```python
from build123d import *

# Parameters (mm, degrees)
SKETCH1_W           = 100
SKETCH1_H           = 40
BOSS_EXTRUDE1_DEPTH = 38
CUT_EXTRUDE2_START  = -12
SKETCH2_W           = 39.5
SKETCH2_H           = 34
CUT_EXTRUDE2_DEPTH  = 21
CUT_EXTRUDE3_DEPTH  = 9
CUT_EXTRUDE4_REACH  = 81.36
SKETCH4_R           = 1.45
SKETCH5_W           = 100
SKETCH5_H           = 19
CUT_EXTRUDE5_DEPTH  = 87.215210375
FILLET1_R           = 0.5
CUT_EXTRUDE11_REACH = 73.063
SKETCH10_R          = 3.5


with BuildPart() as part:
    # Sketch1 → Boss-Extrude1 (new body)
    with BuildSketch(Plane.XY):
        with Locations((16.25, 1.5625)):
            Rectangle(SKETCH1_W, SKETCH1_H)
    extrude(amount=BOSS_EXTRUDE1_DEPTH)

    # Sketch2 → Cut-Extrude2 (cut)
    with BuildSketch(Plane(origin=(0, 0, 0), x_dir=(-1, 0, 0), z_dir=(0, 0, -1)).offset(CUT_EXTRUDE2_START)):
        with Locations((-38.5, 1.5625)):
            Rectangle(SKETCH2_W, SKETCH2_H)
        with Locations((6, 1.5625)):
            Rectangle(SKETCH2_W, SKETCH2_H)
    extrude(amount=-CUT_EXTRUDE2_DEPTH, mode=Mode.SUBTRACT)

    # Sketch3 → Cut-Extrude3 (cut)
    with BuildSketch(Plane(origin=(-3.362318072, 0, 0), x_dir=(-1, 0, 0), z_dir=(0, 0, -1))):
        with BuildLine():
            ThreePointArc((-61.593370612, 1.614325749), (-20.676836723, -17.421621422), (21.715969185, -1.949710178))
            ThreePointArc((21.715969185, -1.949710178), (22.204299442, 9.465009595), (10.78957967, 9.953339852))
            ThreePointArc((10.78957967, 9.953339852), (-19.986233449, -1.278769909), (-49.690320582, 12.540715264))
            ThreePointArc((-49.690320582, 12.540715264), (-61.105040355, 13.029045522), (-61.593370612, 1.614325749))
        make_face()
    extrude(amount=-CUT_EXTRUDE3_DEPTH, mode=Mode.SUBTRACT)

    # Sketch4 → Cut-Extrude4 (cut, up to next)
    with BuildSketch(Plane(origin=(0, 0, 0), x_dir=(-1, 0, 0), z_dir=(0, 0, -1)), mode=Mode.PRIVATE) as cut_extrude4_sk1:
        with Locations((-62.25, 16.0625)):
            Circle(SKETCH4_R)
    cut_extrude4_tool1 = extrude(cut_extrude4_sk1.sketch, amount=-CUT_EXTRUDE4_REACH, mode=Mode.PRIVATE) & part.part
    # Sketch4 → Cut-Extrude4 (cut, up to next)
    with BuildSketch(Plane(origin=(0, 0, 0), x_dir=(-1, 0, 0), z_dir=(0, 0, -1)), mode=Mode.PRIVATE) as cut_extrude4_sk2:
        with Locations((-62.25, -12.9375)):
            Circle(SKETCH4_R)
    cut_extrude4_tool2 = extrude(cut_extrude4_sk2.sketch, amount=-CUT_EXTRUDE4_REACH, mode=Mode.PRIVATE) & part.part
    # Sketch4 → Cut-Extrude4 (cut, up to next)
    with BuildSketch(Plane(origin=(0, 0, 0), x_dir=(-1, 0, 0), z_dir=(0, 0, -1)), mode=Mode.PRIVATE) as cut_extrude4_sk3:
        with Locations((29.75, 16.0625)):
            Circle(SKETCH4_R)
    cut_extrude4_tool3 = extrude(cut_extrude4_sk3.sketch, amount=-CUT_EXTRUDE4_REACH, mode=Mode.PRIVATE) & part.part
    # Sketch4 → Cut-Extrude4 (cut, up to next)
    with BuildSketch(Plane(origin=(0, 0, 0), x_dir=(-1, 0, 0), z_dir=(0, 0, -1)), mode=Mode.PRIVATE) as cut_extrude4_sk4:
        with Locations((29.75, -12.9375)):
            Circle(SKETCH4_R)
    cut_extrude4_tool4 = extrude(cut_extrude4_sk4.sketch, amount=-CUT_EXTRUDE4_REACH, mode=Mode.PRIVATE) & part.part
    add(cut_extrude4_tool1.solids().sort_by_distance((62.25, 16.0625, 0))[0], mode=Mode.SUBTRACT)
    add(cut_extrude4_tool2.solids().sort_by_distance((62.25, -12.9375, 0))[0], mode=Mode.SUBTRACT)
    add(cut_extrude4_tool3.solids().sort_by_distance((-29.75, 16.0625, 0))[0], mode=Mode.SUBTRACT)
    add(cut_extrude4_tool4.solids().sort_by_distance((-29.75, -12.9375, 0))[0], mode=Mode.SUBTRACT)

    # Sketch5 → Cut-Extrude5 (cut, through all)
    with BuildSketch(Plane(origin=(0, 21.5625, 0), x_dir=(1, 0, 0), z_dir=(0, 1, 0))):
        with Locations((16.25, -9.5)):
            Rectangle(SKETCH5_W, SKETCH5_H)
    extrude(amount=-CUT_EXTRUDE5_DEPTH, mode=Mode.SUBTRACT)

    # Fillet1
    fillet1_edges = [part.edges().sort_by_distance(p)[0] for p in [
        (58.25, 18.5625, 26),
        (18.75, 18.5625, 26),
        (18.75, -15.4375, 26),
        (58.25, -15.4375, 26),
        (13.75, 18.5625, 26),
        (-25.75, 18.5625, 26),
        (-25.75, -15.4375, 26),
        (13.75, -15.4375, 26),
    ]]
    fillet(fillet1_edges, radius=FILLET1_R)

    # Sketch10 → Cut-Extrude11 (cut, up to next)
    with BuildSketch(Plane(origin=(0, 0, 33), x_dir=(-1, 0, 0), z_dir=(0, 0, -1)), mode=Mode.PRIVATE) as cut_extrude11_sk1:
        with Locations((-49.860388068, -8.232477434)):
            Circle(SKETCH10_R)
    cut_extrude11_tool1 = extrude(cut_extrude11_sk1.sketch, amount=-CUT_EXTRUDE11_REACH, mode=Mode.PRIVATE) & part.part
    # Sketch10 → Cut-Extrude11 (cut, up to next)
    with BuildSketch(Plane(origin=(0, 0, 33), x_dir=(-1, 0, 0), z_dir=(0, 0, -1)), mode=Mode.PRIVATE) as cut_extrude11_sk2:
        with Locations((-27.139611932, 11.357477434)):
            Circle(SKETCH10_R)
    cut_extrude11_tool2 = extrude(cut_extrude11_sk2.sketch, amount=-CUT_EXTRUDE11_REACH, mode=Mode.PRIVATE) & part.part
    # Sketch10 → Cut-Extrude11 (cut, up to next)
    with BuildSketch(Plane(origin=(0, 0, 33), x_dir=(-1, 0, 0), z_dir=(0, 0, -1)), mode=Mode.PRIVATE) as cut_extrude11_sk3:
        with Locations((-5.360388068, -8.232477434)):
            Circle(SKETCH10_R)
    cut_extrude11_tool3 = extrude(cut_extrude11_sk3.sketch, amount=-CUT_EXTRUDE11_REACH, mode=Mode.PRIVATE) & part.part
    # Sketch10 → Cut-Extrude11 (cut, up to next)
    with BuildSketch(Plane(origin=(0, 0, 33), x_dir=(-1, 0, 0), z_dir=(0, 0, -1)), mode=Mode.PRIVATE) as cut_extrude11_sk4:
        with Locations((17.360388068, 11.357477434)):
            Circle(SKETCH10_R)
    cut_extrude11_tool4 = extrude(cut_extrude11_sk4.sketch, amount=-CUT_EXTRUDE11_REACH, mode=Mode.PRIVATE) & part.part
    add(cut_extrude11_tool1.solids().sort_by_distance((49.860388, -8.232477, 33))[0], mode=Mode.SUBTRACT)
    add(cut_extrude11_tool2.solids().sort_by_distance((27.139612, 11.357477, 33))[0], mode=Mode.SUBTRACT)
    add(cut_extrude11_tool3.solids().sort_by_distance((5.360388, -8.232477, 33))[0], mode=Mode.SUBTRACT)
    add(cut_extrude11_tool4.solids().sort_by_distance((-17.360388, 11.357477, 33))[0], mode=Mode.SUBTRACT)


solid = part.part
```
The model under review builds one solid part; all positions refer to its coordinate system, in mm. A direction names the side the tool comes from. Coordinates: 2 decimals unless noted, no trailing zeros. Write each loop counter-clockwise with the first axis right and the second up, starting at its lowest first coordinate (ties: lowest second). Pieces come first, ordered by that corner, then holes. Notation, with made-up numbers: (63.25, -17) -> (119.25, -17) arc R20 ccw to (119.25, -10) -> close; hole circle Ø2 at (-12, 58.25). An arc over 180 degrees is marked (long way). One line per item, written item: value. Start each with the question number.
Q1. For faces 1 (the face through (-16.6, 7.94, 35.47)), 2 (the face through (18.75, 1, 26)), list the 3-axis set-ups (+Z, -Z, +X, -X, +Y, -Y) from which the entire face can be reached by the end or side of a thin tool; tool diameter is ignored.
Q2. To check wall thickness, follow probe 1 along X at (y, z) = (9.5, 20.25); probe 2 along X at (y, z) = (-13, 21); probe 3 along Y at (x, z) = (62.25, 27.25). State the ranges of each line that lie inside material, in increasing order.
Q3. Add section D-D, the plane z = 22.75. Give the boundary of the cut face in (x, y), then the cut area to 3 significant figures.
Q4. Add section B-B, the plane y = 10. Give the boundary of the cut face in (x, z), then the cut area to 3 significant figures.
Q5. Clearance check with a flat-ended pin moving along its axis: P1, Ø1.5, axis at x = 41.5, y = 10, coming from the -Z side. State where the tip first meets the part, or that it passes through.
Q6. Add section C-C, the plane x = 38.5. Give the boundary of the cut face in (y, z).
Q7. Add section A-A, the plane x = -29.75. Give the boundary of the cut face in (y, z), then the cut area to 3 significant figures.
Q8. The part is to be moulded in two halves that separate along X. For faces 3 (the face through (66.25, 1, 28)), 4 (the face through (16, 2, 19)), 5 (the face through (27.9, 7.94, 35.47)), say which applies: +X half, -X half, draft (parallel to the pull), parting line (faces both ways), or undercut.
Response:
1. face 1: +Z, -Z
1. face 2: -Z
2. probe 1: -33.75 to -25.75, 13.75 to 18.75, 58.25 to 66.25
2. probe 2: -33.75 to -31.2, -28.3 to -25.75, 13.75 to 18.75, 58.25 to 60.8, 63.7 to 66.25
2. probe 3: -18.44 to -14.39, -11.49 to 14.61, 17.51 to 21.56
3. outline: (-33.75, -18.44) -> (66.25, -18.44) -> (66.25, 21.56) -> (-33.75, 21.56) -> close; hole circle Ø2.9 at (-29.75, -12.94); hole circle Ø2.9 at (-29.75, 16.06); hole (-25.75, -14.94) arc R0.5 ccw to (-25.25, -15.44) -> (13.25, -15.44) arc R0.5 ccw to (13.75, -14.94) -> (13.75, 18.06) arc R0.5 ccw to (13.25, 18.56) -> (-25.25, 18.56) arc R0.5 ccw to (-25.75, 18.06) -> close; hole (18.75, -14.94) arc R0.5 ccw to (19.25, -15.44) -> (57.75, -15.44) arc R0.5 ccw to (58.25, -14.94) -> (58.25, 18.06) arc R0.5 ccw to (57.75, 18.56) -> (19.25, 18.56) arc R0.5 ccw to (18.75, 18.06) -> close; hole circle Ø2.9 at (62.25, -12.94); hole circle Ø2.9 at (62.25, 16.06)
3. area: 1,290 mm²
4. outline: (-33.75, 19) -> (-25.75, 19) -> (-25.75, 33) -> (-20.59, 33) -> (-20.59, 38) -> (-33.75, 38) -> close; (-14.13, 33) -> (13.75, 33) -> (13.75, 19) -> (18.75, 19) -> (18.75, 33) -> (23.91, 33) -> (23.91, 38) -> (-14.13, 38) -> close; (30.37, 33) -> (58.25, 33) -> (58.25, 19) -> (66.25, 19) -> (66.25, 38) -> (30.37, 38) -> close
4. area: 729 mm²
5. P1: z = 33
6. outline: (-18.44, 19) -> (-15.44, 19) -> (-15.44, 33) -> (18.56, 33) -> (18.56, 19) -> (21.56, 19) -> (21.56, 38) -> (-18.44, 38) -> close
7. outline: (-18.44, 19) -> (-14.39, 19) -> (-14.39, 38) -> (-18.44, 38) -> close; (-11.49, 19) -> (14.61, 19) -> (14.61, 38) -> (-11.49, 38) -> close; (17.51, 19) -> (21.56, 19) -> (21.56, 38) -> (17.51, 38) -> close
7. area: 650 mm²
8. face 3: +X half
8. face 4: draft
8. face 5: undercut
